Geometry: final body of the model. Coordinates: model frame, mm. Round coordinates to 2 decimals unless told otherwise and drop trailing zeros. Order: outer loops, then holes, each group sorted by start corner. A loop starts at its lowest first (then second) coordinate and runs counter-clockwise, first axis right, second up. Notation, with made-up numbers: (56.5, 13) -> (87.5, 13) arc R11 cw to (87.5, 34) -> close; hole circle Ø1 at (51, 77.5). An arc over 180 degrees is marked (long way). Put each result on its own line as item: value.
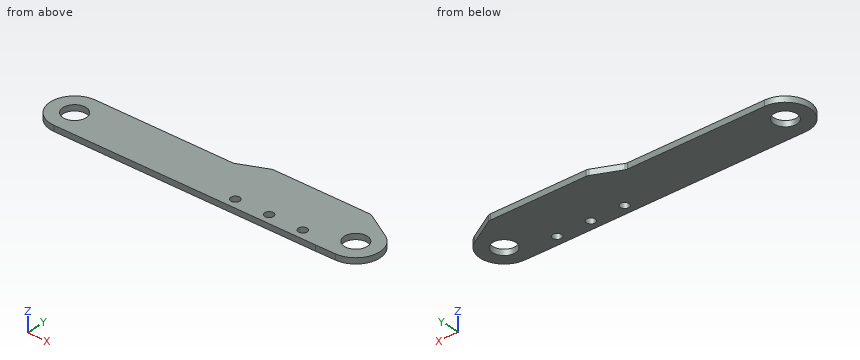
Autodesk Inventor part; units mm, degrees
ref_plane "YZ Plane" through (0, 0, 0) normal (1, 0, 0) x (0, 1, 0)
ref_plane "XZ Plane" through (0, 0, 0) normal (0, 1, 0) x (-1, 0, 0)
ref_plane "XY Plane" through (0, 0, 0) normal (0, 0, 1) x (1, 0, 0)
sketch "スケッチ1" plane through (0, 0, 0) normal (0, 0, 1) x (1, 0, 0)
  line L0 (-50, 0) -> (50, 0) construction
  circle A0 centre (-50, 0) radius 4.05
  circle A1 centre (50, 0) radius 4.05
  line L1 (-50, 8.5) -> (43, 8.5)
  line L2 (-50, -8.5) -> (43, -8.5)
  arc A2 (-50, 8.5) -> (-50, -8.5) centre (-50, 0) ccw
  line L3 (43, -8.5) -> (50.119, -8.3992)
  line L4 (43, 8.5) -> (50.119, 8.3992)
  arc A3 (50.119, -8.3992) -> (50.119, 8.3992) centre (50, 0) ccw
  line L5 (9, -7.5) -> (38, -7.5) construction
  line L6 (38, -7.5) -> (38, -2.5) construction
  line L7 (38, -2.5) -> (9, -2.5) construction
  line L8 (9, -2.5) -> (9, -7.5) construction
  line L9 (9, -5) -> (38, -5) construction
  circle A4 centre (23.5, -5) radius 1.55
  circle A5 centre (11.5, -5) radius 1.55
  circle A6 centre (35.5, -5) radius 1.55
  line L10 (23.5, -5) -> (23.5, -2.5) construction
  line L11 (44.1615, 13) -> (9.1615, 13)
  line L12 (9.1615, 13) -> (-0.8385, 8.5)
  line L13 (44.1615, 13) -> (54.1615, 7.2967)
  point P0 (0, 0)
  point P1 (0, 0)
  point P2 (52.0517, 8.5)
  dimension "d0" = 100
  dimension "d1" = 8.1
  dimension "d2" = 8.5
  dimension "d8" = 8.1
  dimension "d9" = 7
  dimension "d10" = 8.4
  dimension "d12" = 5
  dimension "d13" = 29
  dimension "d14" = 3.1
  dimension "d15" = 2.5
  dimension "d17" = 13
  dimension "d19" = 10
  dimension "d20" = 35
  dimension "d25" = 12
  dimension "d26" = 10
  dimension "d34" = 1
extrude "押し出し1" add sketch "スケッチ1" along normal blind 2
fillet "フィレット1" radius 2 3 edges at (-0.8385, 8.5, 1) (9.1615, 13, 1) (44.1615, 13, 1)
equation "\"d8\" = d1"
equation "\"d19\" = d18"
equation "\"d26\" = d19"
properties part number "リンク_メインフレーム_6_3" material "GFRP"
1. Cut plane B-B on x = 11.5. Return loops of the section in (y, z).
Ans:
outline: (-8.5, 0) -> (-6.55, 0) -> (-6.55, 2) -> (-8.5, 2) -> close; (-3.45, 0) -> (13, 0) -> (13, 2) -> (-3.45, 2) -> close
2. Cut plane D-D on x = 51.5. Return loops of the section in (y, z).
Ans:
outline: (-8.27, 0) -> (-3.76, 0) -> (-3.76, 2) -> (-8.27, 2) -> close; (3.76, 0) -> (8.81, 0) -> (8.81, 2) -> (3.76, 2) -> close
3. Cut plane A-A on y = 0. Return loops of the section in (x, z).
Ans:
outline: (-58.5, 0) -> (-54.05, 0) -> (-54.05, 2) -> (-58.5, 2) -> close; (-45.95, 0) -> (45.95, 0) -> (45.95, 2) -> (-45.95, 2) -> close; (54.05, 0) -> (58.4, 0) -> (58.4, 2) -> (54.05, 2) -> close
4. Contact query for a flat-ended pin moving along its axis: P1, Ø6.5, axis at x = -50, y = 0, coming from the +Z side (1 decimal). Output: stop coordinate, or through.
Ans:
P1: through
5. Cut plane C-C on z = 1.05. Return loops of the section in (x, y).
Ans:
outline: (-50, -8.5) -> (43, -8.5) -> (50.12, -8.4) arc R8.4 ccw to (54.16, 7.3) -> (44.62, 12.74) arc R2 ccw to (43.63, 13) -> (9.59, 13) arc R2 ccw to (8.77, 12.82) -> (-0.45, 8.68) arc R2 cw to (-1.27, 8.5) -> (-50, 8.5) arc R8.5 ccw to start; hole circle Ø8.1 at (-50, 0); hole circle Ø3.1 at (11.5, -5); hole circle Ø3.1 at (23.5, -5); hole circle Ø3.1 at (35.5, -5); hole circle Ø8.1 at (50, 0)
6. Material intervals for probe 1 along Y at (x, z) = (11.5, 1.15); probe 2 along X at (y, z) = (1, 1.65); probe 3 along X at (y, z) = (3.25, 0.95), sorted ascending.
Ans:
probe 1: -8.5 to -6.55, -3.45 to 13
probe 2: -58.44 to -53.92, -46.08 to 46.08, 53.92 to 58.34
probe 3: -57.85 to -52.42, -47.58 to 47.58, 52.42 to 57.75
